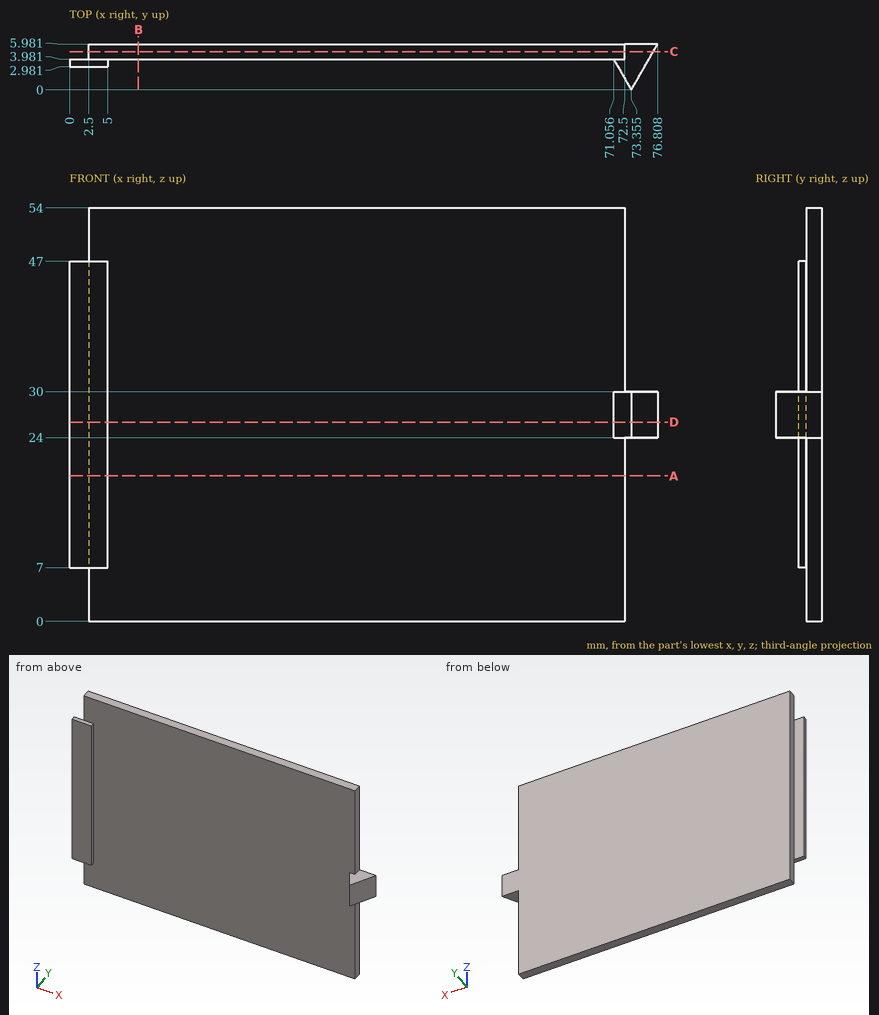
Study the drawing (mm; zero at the part's minimum x, y, z) and answer. Give positions to 0.01 mm unless a question says otherwise; leave off trailing zeros. Write each loop counter-clockwise with the first axis right and the second up, starting at its lowest first coordinate (ties: lowest second). Pieces come first, ordered by that corner, then holes.
(1) The part is cut by section B-B on x = 9. Write down the section's boundary in (y, z), plus the area to 3 significant figures.
Final values:
outline: (3.98, 0) - (5.98, 0) - (5.98, 54) - (3.98, 54) - close
area: 108 mm2
(2) Flat-ended cylindrical pins translate along their axes: pin 1 Ø2 at (y, z) = (5.5, 14.5) entering from -X; pin 2 Ø3 at (x, y) = (73, 2) entering from +Z; pin 3 Ø0.6 at (y, z) = (4.5, 9) entering from +X. Find the tip coordinate at first contact, or state that the pin passes through.
Final values:
pin 1: stops at x = 2.5
pin 2: stops at z = 30
pin 3: stops at x = 72.5
(3) Straight lines are drawn through the part: line 1 (Y direction, x = 54, z = 18.5); line 2 (X direction, y = 5.2, z = 47.5); line 3 (X direction, y = 4.7, z = 24.5). For each, find the intervals that lie inside material, in ascending order.
Final values:
line 1: y = 3.98 to 5.98
line 2: x = 2.5 to 72.5
line 3: x = 2.5 to 76.07
(4) The part is cut by section D-D on z = 26. Write down the section's boundary in (x, y) (1 decimal).
Final values:
outline: (0, 3) - (5, 3) - (5, 4) - (71.1, 4) - (73.4, 0) - (76.8, 6) - (2.5, 6) - (2.5, 4) - (0, 4) - close
(5) The part is cut by section C-C on y = 5. Write down the section's boundary in (x, z), plus the area to 3 significant figures.
Final values:
outline: (2.5, 0) - (72.5, 0) - (72.5, 24) - (76.24, 24) - (76.24, 30) - (72.5, 30) - (72.5, 54) - (2.5, 54) - close
area: 3,800 mm2
(6) The part is cut by section A-A on z = 19. Write down the section's boundary in (x, y), plus the area to 3 significant figures.
Final values:
outline: (0, 2.98) - (5, 2.98) - (5, 3.98) - (72.5, 3.98) - (72.5, 5.98) - (2.5, 5.98) - (2.5, 3.98) - (0, 3.98) - close
area: 145 mm2
